from build123d import *

# Parameters (mm, degrees)
CUT_EXTRUDE1_DEPTH     = 1.85
CUT_EXTRUDE2_START     = -2.85
CUT_EXTRUDE2_OUTLINE_R = 0.9
CUT_EXTRUDE2_DEPTH     = 2.85


# Read off the part's stored shape, not the designer's step: Cut-Extrude2
with BuildPart() as part:
    # Sketch1 → Revolve1 (revolve)
    with BuildSketch(Plane.XY, mode=Mode.PRIVATE) as revolve1_sk:
        Polygon((7.5, 0.9999999999999996), (7.5, 0), (14.000000000000002, 0), (14.000000000000002, 2.8500000000000005), (11.000000000000002, 2.85), (11.000000000000002, 1), align=None)
    revolve(revolve1_sk.sketch.rotate(Axis((3e-17, 0.9999999999999987, 0), (-3e-17, -1, 0)), 180), axis=Axis((3e-17, 0.9999999999999987, 0), (-3e-17, -1, 0)))

    # Sketch2 → Cut-Extrude1 (cut)
    with BuildSketch(Plane(origin=(9e-17, 2.8500000000000005, 0), x_dir=(1, -3e-17, 0), z_dir=(3e-17, 1, 0))):
        with BuildLine():
            ThreePointArc((0.259433716221758, 10.996940217482653), (0.6093823027349546, 10.983107629861117), (0.9587131702244344, 10.958141679009186))
            Line((0.9587131702242476, 10.9581416790092), (1.2201803984672228, 13.946725773284436))
            ThreePointArc((1.2201803984672233, 13.946725773284438), (0.8710215713285331, 13.97287806510457), (0.521317929845157, 13.99029047647053))
            Line((0.5213179298455201, 13.99029047647048), (0.25943371622169603, 10.996940217482662))
        make_face()
        with BuildLine():
            Line((1.2201803984672228, 13.946725773284436), (0.9587131702242476, 10.9581416790092))
            ThreePointArc((0.9587131702244344, 10.958141679009186), (1.3070722087636013, 10.922067672427135), (1.6541062935502489, 10.874922177635916))
            Line((1.6541062935501436, 10.874922177635918), (1.9159905071739696, 13.868272436623787))
            ThreePointArc((1.9159905071740335, 13.868272436623785), (1.5685760162822768, 13.911849958979003), (1.2201803984672233, 13.946725773284438))
        make_face()
        with BuildLine():
            Line((-1.9159905071739802, 13.868272436623787), (-1.654106293550152, 10.874922177635916))
            ThreePointArc((-1.654106293550262, 10.874922177635913), (-0.9587131702243502, 10.958141679009193), (-0.25943371622180056, 10.996940217482653))
            Line((-0.259433716221705, 10.996940217482667), (-0.5213179298455309, 13.990290476470479))
            ThreePointArc((-0.5213179298451552, 13.99029047647053), (-0.8710219940751529, 13.97287803875198), (-1.2201812423779956, 13.946725699451788))
            ThreePointArc((-1.2201812423779956, 13.946725699451788), (-1.5685764371825126, 13.911849911522042), (-1.9159905071740533, 13.868272436623784))
        make_face()
    extrude(amount=-CUT_EXTRUDE1_DEPTH, mode=Mode.SUBTRACT)

    # Cut-Extrude2 outline → Cut-Extrude2 (cut)
    with BuildSketch(Plane(origin=(9e-17, 2.8500000000000005, 0), x_dir=(1, -3e-17, 0), z_dir=(3e-17, 1, 0)).offset(CUT_EXTRUDE2_START)):
        with BuildLine():
            ThreePointArc((8.618451553, 3.35928457), (8.010734985, -4.625), (1.4, -9.143440272))
            Line((1.4, -9.143440272), (1.4, -13.929824119))
            ThreePointArc((1.4, -13.929824119), (12.124355653, -7), (12.763581558, 5.752476494))
            Line((12.763581558, 5.752476494), (8.618451553, 3.35928457))
        make_face()
        with BuildLine():
            Line((-8.618451553, 3.35928457), (-12.763581558, 5.752476494))
            ThreePointArc((-12.763581558, 5.752476494), (-12.124355653, -7), (-1.4, -13.929824119))
            Line((-1.4, -13.929824119), (-1.4, -9.143440272))
            ThreePointArc((-1.4, -9.143440272), (-8.010734985, -4.625), (-8.618451553, 3.35928457))
        make_face()
        with BuildLine():
            Line((2.5, 13.774977314), (2.5, 8.905756565))
            ThreePointArc((2.5, 8.905756565), (5.103741092, 7.714552927), (7.218451553, 5.784155701))
            Line((7.218451553, 5.784155701), (11.363581558, 8.177347625))
            ThreePointArc((11.363581558, 8.177347625), (7.475499176, 11.837098972), (2.5, 13.774977314))
        make_face()
        with BuildLine():
            Line((-2.5, 8.905756565), (-2.5, 13.774977314))
            ThreePointArc((-2.5, 13.774977314), (-7.475499176, 11.837098972), (-11.363581558, 8.177347625))
            Line((-11.363581558, 8.177347625), (-7.218451553, 5.784155701))
            ThreePointArc((-7.218451553, 5.784155701), (-5.103741092, 7.714552927), (-2.5, 8.905756565))
        make_face()
        with Locations((-10.825317547, 6.25)):
            Circle(CUT_EXTRUDE2_OUTLINE_R)
        with Locations((0, -12.5)):
            Circle(CUT_EXTRUDE2_OUTLINE_R)
        with Locations((10.825317547, 6.25)):
            Circle(CUT_EXTRUDE2_OUTLINE_R)
    extrude(amount=CUT_EXTRUDE2_DEPTH, mode=Mode.SUBTRACT)


solid = part.part
CAD build for the part. Positions are in the model's coordinates, mm. A direction names the side the tool comes from. Coordinates: 2 decimals unless noted, no trailing zeros. Loops run counter-clockwise (first coordinate to the right, second up) from the corner with the lowest first, then second, coordinate; pieces in that order, holes last. Notation, with made-up numbers: (16.5, 37.5) - (55.5, 37.5) arc R26 cw to (55.5, 75.5) - close; hole circle Ø5 at (12.5, -32.5). An arc over 180 degrees is marked (long way). Use one line per item in the form item = value. Start each with the question number.
1) Band-saw the part on D-D (z = -6.25). Give the cut face in (x, y), and give its area (3 significant figures).
2) Flat gauge pins, fed straight in: pin 1 (1 mm diameter, centred on x = -7.5, y = 0.5, fed in from +Z); pin 2 (4 mm diameter, centred on x = 7.5, z = 0, fed in from +Y); pin 3 (0.9 mm diameter, centred on y = 1.5, z = 12.5, fed in from -X); pin 4 (1.5 mm diameter, centred on x = -3.5, z = -4.5, fed in from +Y). Where does each tip first touch, or does it go through?
3) Drill centre lines: L1, parallel to Z at x = 0, y = 0.6; L2, parallel to Z at x = 0, y = 1.5; L3, parallel to X at y = 2.45, z = -7. Where is each one in solid material? Low to high. Write a range as from..to.
4) Band-saw the part on B-B (z = 0). Give the cut face in (x, y).
5) Band-saw the part on C-C (x = -5). Give the cut face in (y, z).
6) Tool access for faces 1 (the face through (-1.4, 1, 12)), 2 (the face through (2.5, 1, -12)), 3 (the face through (-9.54, 1.91, -5.48)): list every direction of +Z, -Z, +X, -X, +Y, -Y with a clear straight run to the whole face (end or side of a thin tool).
7) Two-plate mould, pull along Z, no slides. Class faces 4 (the face through (9.926, 1.405, -6.29)), 5 (the face through (-2, 2.85, -12)), 6 (the face through (-2.08, 1.91, -10.8)): +Z half, -Z half, draft (parallel to the pull), parting line (faces both ways), or undercut.
8) Band-saw the part on A-A (y = 1.5). State how many separate pieces and enclosed holes the cut face has, and give its area (3 significant figures).
Check values:
q1.outline = (-12.53, 0) - (-11.73, 0) - (-11.73, 2.85) - (-12.53, 2.85) - close; (-9.93, 0) - (-8.03, 0) - (-8.03, 1) - (-9.05, 1) - (-9.05, 2.85) - (-9.93, 2.85) - close; (-6.82, 0) - (-4.15, 0) - (-4.15, 1) - (-6.82, 1) - close; (4.15, 0) - (6.82, 0) - (6.82, 1) - (4.15, 1) - close; (8.03, 0) - (9.93, 0) - (9.93, 2.85) - (9.05, 2.85) - (9.05, 1) - (8.03, 1) - close; (11.73, 0) - (12.53, 0) - (12.53, 2.85) - (11.73, 2.85) - close
q1.area = 17.0 mm2
q2.pin_1 = 6.05
q2.pin_2 = 1
q2.pin_3 = -1.4
q2.pin_4 = through
q3.L1 = -14..-7.5, 7.5..11.6, 13.4..14
q3.L2 = -14..-11, 11..11.6, 13.4..14
q3.L3 = -12.12..-11.32, -10.33..-9.32, 9.32..10.33, 11.32..12.12
q4.outline = (-9.25, 0) - (-7.5, 0) - (-7.5, 1) - (-9.25, 1) - close; (7.5, 0) - (9.25, 0) - (9.25, 1) - (7.5, 1) - close
q5.outline = (0, -7.78) - (1, -7.78) - (1, -5.59) - (0, -5.59) - close; (0, 5.59) - (1, 5.59) - (1, 7.78) - (0, 7.78) - close
q6.face_1 = +Z, -X, +Y, -Y
q6.face_2 = -Z, +X, +Y, -Y
q6.face_3 = +Z, +Y
q7.face_4 = undercut
q7.face_5 = draft
q7.face_6 = +Z half
q8.separate_pieces = 6
q8.enclosed_holes = 3
q8.area = 24.3 mm2
